Geometry: final body of the model. Coordinates: model frame, mm. A direction names the side the tool comes from. Coordinates: 2 decimals unless noted, no trailing zeros. Put each result on its own line as item: value.
```python
from build123d import *

# Parameters (mm, degrees)
SKETCH_1_R               = 50
SKETCH_1_R_2             = 1.75
SKETCH_1_R_3             = 5
EXTRUDE_1_DEPTH          = 5
SKETCH_2_R               = 1.5
CUT_EXTRUDE_1_DEPTH      = 2
SKETCH_3_R               = 3
SKETCH_2_3_R             = 1.5
CUT_EXTRUDE_2_DEPTH      = 1
CUT_EXTRUDE_2_DEPTH_BACK = 6
SKETCH_4_R               = 1.75
SKETCH_4_R_2             = 3
SKETCH_4_R_3             = 1.5
CUT_EXTRUDE_3_DEPTH      = 2


with BuildPart() as part:
    # Эскиз1 → Бобышка-Вытянуть1 (new body)
    with BuildSketch(Plane(origin=(0, 0, 0), x_dir=(1, 0, 0), z_dir=(0, 1, 0))):
        Circle(SKETCH_1_R)
        with Locations((-23.5, 13)):
            Circle(SKETCH_1_R_2, mode=Mode.SUBTRACT)
        with Locations((-23.5, -13)):
            Circle(SKETCH_1_R_2, mode=Mode.SUBTRACT)
        Circle(SKETCH_1_R_3, mode=Mode.SUBTRACT)
        with Locations((23.5, -13)):
            Circle(SKETCH_1_R_2, mode=Mode.SUBTRACT)
        with Locations((23.5, 13)):
            Circle(SKETCH_1_R_2, mode=Mode.SUBTRACT)
    extrude(amount=EXTRUDE_1_DEPTH)

    # Эскиз2 → Вырез-Вытянуть1 (cut)
    with BuildSketch(Plane.XZ):
        with Locations((0, 13.5)):
            Circle(SKETCH_2_R)
        with Locations((11.691342951, 6.75)):
            Circle(SKETCH_2_R)
        with Locations((11.691342951, -6.75)):
            Circle(SKETCH_2_R)
        with Locations((0, -13.5)):
            Circle(SKETCH_2_R)
        with Locations((-11.691342951, -6.75)):
            Circle(SKETCH_2_R)
        with Locations((-11.691342951, 6.75)):
            Circle(SKETCH_2_R)
        Polygon((-25.232050808, 16), (-26.964101615, 13), (-25.232050808, 10), (-21.767949192, 10), (-20.035898385, 13), (-21.767949192, 16), align=None)
        Polygon((21.767949192, 16), (20.035898385, 13), (21.767949192, 10), (25.232050808, 10), (26.964101615, 13), (25.232050808, 16), align=None)
        Polygon((21.767949192, -10), (20.035898385, -13), (21.767949192, -16), (25.232050808, -16), (26.964101615, -13), (25.232050808, -10), align=None)
        Polygon((-25.232050808, -10), (-26.964101615, -13), (-25.232050808, -16), (-21.767949192, -16), (-20.035898385, -13), (-21.767949192, -10), align=None)
    extrude(amount=-CUT_EXTRUDE_1_DEPTH, mode=Mode.SUBTRACT)

    # Эскиз3 → Вырез-Повернуть1 (revolve, cut)
    with BuildSketch(Plane.XY):
        with Locations((-45, -1.5)):
            Circle(SKETCH_3_R)
    revolve(axis=Axis((0, 0, 0), (0, -1, 0)), mode=Mode.SUBTRACT)

    # Эскиз2<3> → Вырез-Вытянуть2 (cut, two sides)
    with BuildSketch(Plane.XZ) as cut_extrude_2_sk:
        with Locations((0, -13.5)):
            Circle(SKETCH_2_3_R)
        with Locations((-11.691342951, -6.75)):
            Circle(SKETCH_2_3_R)
        with Locations((-11.691342951, 6.75)):
            Circle(SKETCH_2_3_R)
        with Locations((11.691342951, -6.75)):
            Circle(SKETCH_2_3_R)
        with Locations((0, 13.5)):
            Circle(SKETCH_2_3_R)
        with Locations((11.691342951, 6.75)):
            Circle(SKETCH_2_3_R)
    extrude(amount=CUT_EXTRUDE_2_DEPTH, mode=Mode.SUBTRACT)
    extrude(cut_extrude_2_sk.sketch, amount=-CUT_EXTRUDE_2_DEPTH_BACK, mode=Mode.SUBTRACT)

    # Эскиз4 → Вырез-Вытянуть3 (cut)
    with BuildSketch(Plane(origin=(0, 5, 0), x_dir=(1, 0, 0), z_dir=(0, 1, 0))):
        with Locations((-23.5, -13)):
            Circle(SKETCH_4_R)
        with Locations((-11.691342951, 6.75)):
            Circle(SKETCH_4_R_2)
        with Locations((-11.691342951, 6.75)):
            Circle(SKETCH_4_R_3, mode=Mode.SUBTRACT)
        with Locations((0, 13.5)):
            Circle(SKETCH_4_R_2)
        with Locations((0, 13.5)):
            Circle(SKETCH_4_R_3, mode=Mode.SUBTRACT)
        with Locations((11.691342951, 6.75)):
            Circle(SKETCH_4_R_2)
        with Locations((11.691342951, -6.75)):
            Circle(SKETCH_4_R_2)
        with Locations((0, -13.5)):
            Circle(SKETCH_4_R_2)
        with Locations((-11.691342951, -6.75)):
            Circle(SKETCH_4_R_2)
    extrude(amount=-CUT_EXTRUDE_3_DEPTH, mode=Mode.SUBTRACT)


solid = part.part
```
1. Pin query (flat end, axial travel): pin 1 Ø1 at (x, y) = (23, 1) entering from -Z; pin 2 Ø1.8 at (x, z) = (1.5, -12.5) entering from +Y; pin 3 Ø2 at (x, y) = (23, 1) entering from -Z. Return the tip coordinate at first contact, or that it passes through.
Answer below:
pin 1: stops at z = -44.65
pin 2: stops at y = 3
pin 3: stops at z = -44.9
2. Section query A-A (z = 6.75). Count the separate pieces of the cut face and the enclosed holes in it, then the cut area to 3 significant figures.
Answer below:
separate pieces: 3
enclosed holes: 0
area: 442 mm²
3. Set-up query: faces 1 (the flat face through (10, 3, -6)), 2 (the cylindrical face through (0, 1, 12)), 3 (the flat face through (-22, 2, -14.3)). Return all of +Z, -Z, +X, -X, +Y, -Y with unobstructed straight access to the full face (end or side cutting, diameter ignored); none if empty.
Answer below:
face 1: +Y
face 2: +Y, -Y
face 3: -Y
4. Ray query, probe 1 along Z at (x, y) = (0, 4.05); probe 2 along Z at (x, y) = (0, 0.8); probe 3 along Z at (x, y) = (23.5, 3.5). Return the intervals inside material, ascending. Write a range as from..to.
Answer below:
probe 1: z = -50..-16.5, -10.5..-5, 5..10.5, 16.5..50
probe 2: z = -50..-46.93, -43.07..-15, -12..-5, 5..12, 15..43.07, 46.93..50
probe 3: z = -44.13..-14.75, -11.25..11.25, 14.75..44.13
5. Mould query, pull axis X, two halves, no side actions, for faces 4 (the flat face through (44.2, 0, 18.3)), 5 (the cylindrical face through (47.69, 2.46, -15.02)), 6 (the cylindrical face through (-0.65, 4.01, -10.57)). Classes: +X half, -X half, draft (parallel to the pull), parting line (faces both ways), or undercut.
Answer below:
face 4: draft
face 5: parting line
face 6: undercut
